from build123d import *

# Parameters (mm, degrees)
F0_W     = 50.8
F0_H     = 12.7
F1_DEPTH = 31.75
F3_DEPTH = 12.7
F4_W     = 12.7
F4_H     = 19.05
F5_DEPTH = 19.05
F6_DEPTH = 19.05
F8_DEPTH = 50.8


with BuildPart() as f1:
    # F0 (on Front) → F1 (new body)
    with BuildSketch(Plane.XZ):
        with Locations((25.4, 6.35)):
            Rectangle(F0_W, F0_H)
    extrude(amount=F1_DEPTH)

    # F2 (on Front) → F3 (join)
    with BuildSketch(Plane.XZ):
        Polygon((0, 12.135556), (50.79918, 12.424188), (38.1, 31.185556), (0, 31.185556), align=None)
    extrude(amount=F3_DEPTH)

    # F4 (on face) → F5 (join)
    with BuildSketch(Plane.XY.offset(12.7)):
        with Locations((25.4, -22.225)):
            Rectangle(F4_W, F4_H)
    extrude(amount=F5_DEPTH)

    # F4 (on face) → F6 (join)
    with BuildSketch(Plane.XY.offset(12.7)):
        with Locations((25.4, -22.225)):
            Rectangle(F4_W, F4_H)
    extrude(amount=F6_DEPTH)

    # F7 (on face) → F8 (cut)
    with BuildSketch(Plane.YZ.offset(31.75)):
        Polygon((-31.75, 12.7), (-12.7, 31.75), (-31.75, 31.75), align=None)
    extrude(amount=-F8_DEPTH, mode=Mode.SUBTRACT)


solid = f1.part
Here's how the part is built. I have some questions about the finished solid (model axes, mm). A direction names the side the tool comes from. Give positions to 0.01 mm unless a question says otherwise; leave off trailing zeros. Write each loop counter-clockwise with the first axis right and the second up, starting at its lowest first coordinate (ties: lowest second). Pieces come first, ordered by that corner, then holes. Notation, with made-up numbers: (53, 82.25) -> (90, 82.25) arc R25 ccw to (90, 107.25) -> close; hole circle Ø11 at (88, 43.25). An arc over 180 degrees is marked (long way). Use one line per item in the form item = value. Start each with the question number.
1. If I drill on L1, parallel to Z at x = 34, y = -15; L2, parallel to Y at x = 35, z = 27.5; L3, parallel to X at y = -20, z = 14, over which ranges is the centre line in solid material (lowest first)?
2. Imagine slicing it at B-B on z = 29. List the corners of the cut face in (x, y) for me.
3. On a 3-axis mill with a long thin cutter (end or side, diameter ignored), from which of +Z, -Z, +X, -X, +Y, -Y can I reach the whole of each face in a straight line? I mean faces 1 (the face through (19, -6, 31.186)), 2 (the face through (25.49, -22.36, 22.09)), 3 (the face through (0, -12, 12)), 4 (the face through (9, -22, 12.7)), 5 (the face through (41, -23, 12.7)). Say none if no direction works.
4. Will these pins go through, and if not, where does the flat tip stop? pin 1 Ø15 at (x, z) = (5.5, 22.5) entering from -Y; pin 2 Ø8 at (x, y) = (17.5, -3.5) entering from +Z; pin 3 Ø12 at (x, z) = (14.5, 18) entering from -Y; pin 4 Ø15 at (y, z) = (-25, 23) entering from -X.
5. Imagine slicing it at A-A on y = -27. List the corners of the cut face in (x, z) for me, plus the area to 3 significant figures.
6. Imagine slicing it at D-D on x = 21.5. List the corners of the cut face in (y, z) for me, plus the area to 3 significant figures.
7. Imagine slicing it at C-C on x = 8. List the corners of the cut face in (y, z) for me, plus the area to 3 significant figures.
Entries:
q1.L1 = 0 to 12.7
q1.L2 = -12.7 to 0
q1.L3 = 19.05 to 31.75
q2.outline = (0, -12.7) -> (19.05, -12.7) -> (19.05, -15.45) -> (31.75, -15.45) -> (31.75, -12.7) -> (39.58, -12.7) -> (39.58, 0) -> (0, 0) -> close
q3.face_1 = +Z, +X, -X, +Y
q3.face_2 = +Z, +X, -X, -Y
q3.face_3 = +Z, -Z, -X, +Y, -Y
q3.face_4 = +Z, -X, -Y
q3.face_5 = +Z, +X, -Y
q4.pin_1 = -12.7
q4.pin_2 = 31.19
q4.pin_3 = -31.75
q4.pin_4 = 19.05
q5.outline = (0, 0) -> (50.8, 0) -> (50.8, 12.7) -> (31.75, 12.7) -> (31.75, 17.45) -> (19.05, 17.45) -> (19.05, 12.7) -> (0, 12.7) -> close
q5.area = 705 mm²
q6.outline = (-31.75, 0) -> (0, 0) -> (0, 31.19) -> (-12.7, 31.19) -> (-12.7, 31.75) -> (-31.75, 12.7) -> close
q6.area = 819 mm²
q7.outline = (-31.75, 0) -> (0, 0) -> (0, 31.19) -> (-12.7, 31.19) -> (-12.7, 12.7) -> (-31.75, 12.7) -> close
q7.area = 638 mm²
